Can you work these out from the model? Positions are in its coordinate system, mm. A direction names the side the tool comes from. Round coordinates to 2 decimals unless told otherwise and drop trailing zeros. Loops run counter-clockwise (first coordinate to the right, second up) from the corner with the lowest first, then second, coordinate; pieces in that order, holes last. Notation, with made-up numbers: M 74,-2.5 L 91,-2.5 A8 cw 91,7.5 Z; hole C 74.5,22 d7. An arc over 180 degrees is marked long. Answer as CSV lines item,"result".
Autodesk Inventor part; units mm, degrees
ref_plane "YZ Plane" through (0, 0, 0) normal (1, 0, 0) x (0, 1, 0)
ref_plane "XZ Plane" through (0, 0, 0) normal (0, 1, 0) x (-1, 0, 0)
ref_plane "XY Plane" through (0, 0, 0) normal (0, 0, 1) x (1, 0, 0)
sketch "Sketch1" plane through (0, 0, 0) normal (0, 1, 0) x (-1, 0, 0)
  line L0 (-25.8445, -28.2321) -> (25.8445, -28.2321) construction
  line L1 (25.8445, -28.2321) -> (25.8445, 28.2321) construction
  line L2 (25.8445, 28.2321) -> (-25.8445, 28.2321) construction
  line L3 (-25.8445, 28.2321) -> (-25.8445, -28.2321) construction
  line L4 (-25.8445, -28.2321) -> (25.8445, 28.2321) construction
  line L5 (25.8445, -28.2321) -> (-25.8445, 28.2321) construction
  circle A0 centre (0, 0) radius 28.2321 construction
  arc A1 (-25.8445, -11.3628) -> (0, -28.2321) centre (0, 0) ccw
  arc A2 (25.8445, 11.3628) -> (0, 28.2321) centre (0, 0) ccw
  line L6 (25.8445, 11.3628) -> (25.8445, -28.2321)
  line L7 (25.8445, -28.2321) -> (0, -28.2321)
  line L8 (-25.8445, -11.3628) -> (-25.8445, 28.2321)
  line L9 (-25.8445, 28.2321) -> (0, 28.2321)
  dimension "d2" = 51.689
  dimension "d3" = 56.4642
extrude "Extrusion1" add sketch "Sketch1" along normal blind 89.4842
sketch "Sketch2" plane through (0, 0, 0) normal (0, -1, 0) x (1, 0, 0)
  circle A0 centre (0, 0) radius 8.89
  dimension "d6" = 17.78
extrude "Extrusion2" add sketch "Sketch2" along normal blind 48.26
sketch "Sketch3" plane through (0, 0, 0) normal (0, 0, 1) x (1, 0, 0)
  line L0 (-8.89, -48.26) -> (8.89, -48.26)
  line L1 (8.89, 0) -> (-8.89, 0)
  line L2 (0, -48.26) -> (0, -25.4) construction
  line L3 (0, -25.4) -> (18.288, -25.4) construction
  circle A0 centre (18.288, -25.4) radius 18.288
  dimension "d9" = 22.86
  dimension "d10" = 18.288
extrude "Extrusion3" add sketch "Sketch3" along normal blind 9.144 and the other way blind 9.144
sketch "Sketch4" plane through (18.288, -25.4, 9.144) normal (0, 0, 1) x (1, 0, 0)
  circle A0 centre (0, 0) radius 8.001
  dimension "d15" = 16.002
extrude "Extrusion4" add sketch "Sketch4" along normal blind 17.145
mirror "Mirror1" about plane through (0, 0, 0) normal (0, 0, 1) of "Extrusion4"
sketch "Sketch5" plane through (0, 89.4842, 0) normal (0, 1, 0) x (1, 0, 0)
  arc A0 (25.8445, 11.3628) -> (0, 28.2321) centre (0, 0) ccw construction
  line L0 (25.8445, -28.2321) -> (25.8445, 11.3628) construction
  line L1 (25.8445, 11.3628) -> (35.184, 20.7023)
  line L2 (25.8445, 11.3628) -> (39.0525, 11.3628) construction
  line L3 (35.184, 20.7023) -> (20.4563, 35.4299)
  line L4 (20.4563, 35.4299) -> (11.0193, 25.9928)
  arc A1 (25.8445, 11.3628) -> (11.0193, 25.9928) centre (0, 0) ccw
  dimension "d18" = 13.208
  dimension "d19" = 45
  dimension "d20" = 20.828
extrude "Extrusion5" add sketch "Sketch5" against normal blind 15.24
properties part number "Motor_500RPM" material "Aluminum 6061"
Item 1: If we section it at B-B on z = -16.5: Write out the boundary of the cut face in (x, y), then the cut area to 3 significant figures.
Output:
outline,"M -25.84,0 L 22.91,0 L 22.91,74.24 L 30.98,74.24 L 30.98,89.48 L -25.84,89.48 Z; C 18.29,-25.4 d16"
area,"4,690 mm2"
Item 2: We'd pull the mould along Y, two halves only. Please class faces 5 (the face through (13, 44, 28.232)), 6 (the face through (23, 74.244, -24)), 7 (the face through (0, -48.26, 0)): released by +Y, released by -Y, zero draft, split by the parting line, or undercut.
Output:
face 5,"zero draft"
face 6,"undercut"
face 7,"released by -Y"
Item 3: Will these pins go through, and if not, where does the flat tip stop? pin 1 (5 mm diameter, centred on x = -14, y = 55.5, fed in from +Z); pin 2 (12 mm diameter, centred on y = 58.5, z = 12.5, fed in from +X); pin 3 (5 mm diameter, centred on x = 18.5, y = -26.5, fed in from -Z).
Output:
pin 1,"stops at z = 25.78"
pin 2,"stops at x = 25.84"
pin 3,"stops at z = -26.29"
Item 4: On a 3-axis mill with a long thin cutter (end or side, diameter ignored), from which of +Z, -Z, +X, -X, +Y, -Y can I reach the whole of each face in a straight line? I mean faces 1 (the face through (10.295, -25.048, -17.596)), 2 (the face through (11.94, -20.53, 17.6)), 3 (the face through (18, -25, 26.289)), 4 (the face through (6, 0, 7)). Say none if no direction works.
Output:
face 1,"-Z"
face 2,"+Z"
face 3,"+Z, +X, -X, -Y"
face 4,"none"
Item 5: If I drill on line 1 along Y through (x, z) = (19, 4.5); line 2 along X through (y, z) = (62.5, -9.5); line 3 along Y through (x, z) = (25.5, 16), over which ranges is the centre line in solid material (lowest first)? Write a range as from..to.
Output:
line 1,"y = -43.67..-7.13, 0..89.48"
line 2,"x = -25.84..25.84"
line 3,"y = -28.86..-21.94, 0..89.48"
Item 6: If we section it at A-A on x = 33.5: Write out the boundary of the cut face in (y, z), then the cut area to 3 significant figures.
Output:
outline,"M -35.55,-9.14 L -15.25,-9.14 L -15.25,9.14 L -35.55,9.14 Z; M 74.24,-22.39 L 89.48,-22.39 L 89.48,-19.02 L 74.24,-19.02 Z"
area,"423 mm2"
Item 7: If we section it at C-C on y = 37: Write out the boundary of the cut face in (x, z).
Output:
outline,"M -25.84,-28.23 L 0,-28.23 A28.23 ccw 25.84,-11.36 L 25.84,28.23 L 0,28.23 A28.23 ccw -25.84,11.36 Z"
Item 8: If we section it at D-D on z = -7.5: Write out the boundary of the cut face in (x, y).
Output:
outline,"M -25.84,0 L -4.77,0 L -4.77,-48.26 L 4.77,-48.26 L 4.77,-37.72 A18.29 ccw long 4.77,-13.08 L 4.77,0 L 25.84,0 L 25.84,89.48 L -25.84,89.48 Z"
